Autodesk Fusion 360 part; units mm, degrees
sketch "Sketch1" plane through (0, 0, 0) normal (0, 0, 1) x (1, 0, 0)
  line L0 (0, 0) -> (7, 0)
  line L1 (7, 0) -> (7, 7)
  line L2 (7, 7) -> (0, 7)
  line L3 (0, 7) -> (0, 0)
  line L4 (7, 0) -> (29.8, 0)
  line L5 (29.8, 0) -> (29.8, 7)
  line L6 (29.8, 7) -> (7, 7)
  line L7 (7, 7) -> (7, 0)
  line L8 (29.8, 0) -> (36.8, 0)
  line L9 (36.8, 0) -> (36.8, 7)
  line L10 (36.8, 7) -> (29.8, 7)
  line L11 (29.8, 7) -> (29.8, 0)
  line L12 (0, 7) -> (7, 0)
  line L13 (0, 0) -> (7, 7)
  line L14 (29.8, 7) -> (36.8, 0)
  line L15 (29.8, 0) -> (36.8, 7)
  circle A0 centre (3.5, 3.5) radius 2.3
  circle A1 centre (33.3, 3.5) radius 2.3
  circle A2 centre (3.5, 3.5) radius 3.5
  circle A3 centre (33.3, 3.5) radius 3.5128
  circle A4 centre (33.3, 3.5) radius 3
  circle A5 centre (3.5, 3.5) radius 3
  line L16 (29.8, 7) -> (7, 0)
  line L17 (29.8, 0) -> (7, 7)
  line L18 (7.9, 1) -> (28.9, 1)
  line L19 (28.9, 1) -> (28.9, 6)
  line L20 (28.9, 6) -> (7.9, 6)
  line L21 (7.9, 6) -> (7.9, 1)
  line L22 (7.9, 1) -> (28.9, 6) construction
  line L23 (28.9, 1) -> (7.9, 6) construction
  point P0 (18.4, 3.5)
  dimension "d1" = 7
  dimension "d2" = 7
  dimension "d3" = 22.8
  dimension "d4" = 7
  dimension "d5" = 4.6
  dimension "d6" = 4.6
  dimension "d9" = 6
  dimension "d10" = 6
  dimension "d13" = 21
  dimension "d14" = 5
extrude "Extrude1" add sketch "Sketch1" along normal blind 5 contours L0 L12 A2 | L12 L13 A2 A5 | L12 L13 A2 A5 | L1 L7 L12 A2 | L4 L16 L17 L18 | L1 L7 L16 L17 L18 L20 L21 | L12 L13 A2 A5 | L12 L13 A2 A5 | L12 L13 A0 A5 | L12 L13 A0 A5 | L1 L7 L13 A2 | L5 L11 A3 L16 L17 L18 L19 L20 | L8 L15 A3 | L5 L11 L15 A3 | L16 L17 L18 L20 L21 | L16 L17 L18 | L12 L13 A0 A5 | L2 L13 A2 | L12 L13 A0 A5 | L6 L16 L17 L20 | L5 L11 L14 L15 A3 A4 | L8 L14 L15 A3 A4 | L16 L17 L18 L19 L20 | L16 L17 L20 | L5 L11 L14 A3 | L10 L14 A3 | L14 L15 A1 A4 | L14 L15 A1 A4 | L10 L14 L15 A3 A4 | L9 L14 L15 A3 A4 | L14 L15 A1 A4 | L14 L15 A1 A4
extrude "Extrude2" cut sketch "Sketch1" along normal blind 3.5 contours L12 L13 A0 A5 | L12 L13 A0 A5 | L12 L13 A0 A5 | L12 L13 A0 A5 | L14 L15 A1 A4 | L14 L15 A1 A4 | L14 L15 A1 A4 | L14 L15 A1 A4
extrude "Extrude3" add sketch "Sketch1" along normal blind 8 contours L16 L17 L18 L20 L21 | L16 L17 L18 | L16 L17 L18 L19 L20 | L16 L17 L20
fillet "Fillet1" radius 1.5 1 edges at (7.9, 6, 6.5)
fillet "Fillet2" radius 1.5 1 edges at (7.9, 1, 6.5)
fillet "Fillet3" radius 1.5 1 edges at (28.9, 6, 6.5)
fillet "Fillet4" radius 1.5 1 edges at (28.9, 1, 6.5)
Source: CAD feature listing. Evaluate the final solid. Frame: model axes, mm. A direction names the side the tool comes from. Give positions to 0.01 mm unless a question says otherwise; leave off trailing zeros. Loops run counter-clockwise (first coordinate to the right, second up) from the corner with the lowest first, then second, coordinate; pieces in that order, holes last. Notation, with made-up numbers: (48.25, 32) -> (78.25, 32) arc R27 cw to (78.25, 52) -> close; hole circle Ø1 at (-8, -20.5). An arc over 180 degrees is marked (long way). Use a Markdown table: item, result. Add a question column.
1) Section query B-B, the plane z = 0.75. Return the cut outline in (x, y).
2) Pull-direction query (Y, two-part tool) for faces 1 (the face through (28.45, 1.43, 6.52)), 2 (the face through (35.76, 6.01, 2.46)), 3 (the face through (35.425, 4.381, 4.24)), 4 (the face through (7.9, 4, 6)); classes: +Y half, -Y half, draft (parallel to the pull), parting line (faces both ways), or undercut.
3) Section query D-D, the plane x = 18.5. Return the cut outline in (y, z).
4) Section query C-C, the plane y = 5.25. Return the cut outline in (x, z), then the cut area to 3 significant figures.
5) First-contact query: pin 1 (3.5 mm diameter, centred on x = 3.5, y = 3.5, fed in from -Z); pin 2 (2.5 mm diameter, centred on x = 20, z = 7, fed in from +Y); pin 3 (0.9 mm diameter, centred on x = 21, z = 7, fed in from -Y); pin 4 (1.6 mm diameter, centred on y = 3.5, z = 6, fed in from +X). Flat tips, straight axial feed; report the tip coordinate or a pass-through.
6) Reachability of faces 5 (the face through (0.5, 3.4, 1.7)), 6 (the face through (28.47, 5.55, 6.52)), 7 (the face through (8.33, 1.45, 6.52)), 8 (the face through (8.35, 5.57, 6.52)) from +Z, -Z, +X, -X, +Y, -Y: full face, straight path, thin tool, end or side. Return the list, or none.
7) Section query A-A, the plane x = 5. Return the cut outline in (y, z).
8) Line query: line 1 along Y through (x, z) = (3.5, 1.4); line 2 along X through (y, z) = (1.25, 3); line 3 along X through (y, z) = (1, 1). Output: solid intervals per line, ascending. Write a range as [from, to].
Numbers:
| question | item | result |
|---|---|---|
| 1 | outline | (3.5, 0) -> (33.6, 0) arc R3.51 ccw to (36.8, 3.2) -> (36.8, 3.8) arc R3.51 ccw to (33.6, 7) -> (3.5, 7) arc R3.5 ccw to start; hole circle Ø6 at (3.5, 3.5); hole (29.8, 3.2) -> (29.8, 3.8) arc R3.51 ccw to start; hole circle Ø6 at (33.3, 3.5) |
| 2 | face 1 | -Y half |
| 2 | face 2 | +Y half |
| 2 | face 3 | undercut |
| 2 | face 4 | draft |
| 3 | outline | (0, 0) -> (7, 0) -> (7, 5) -> (6, 5) -> (6, 8) -> (1, 8) -> (1, 5) -> (0, 5) -> close |
| 4 | outline | (0.47, 0) -> (1.06, 0) -> (1.06, 3.5) -> (2.01, 3.5) -> (2.01, 5) -> (0.47, 5) -> close; (4.99, 3.5) -> (5.94, 3.5) -> (5.94, 0) -> (30.86, 0) -> (30.86, 3.5) -> (31.81, 3.5) -> (31.81, 5) -> (28.7, 5) -> (28.7, 8) -> (8.1, 8) -> (8.1, 5) -> (4.99, 5) -> close; (34.79, 3.5) -> (35.74, 3.5) -> (35.74, 0) -> (36.35, 0) -> (36.35, 5) -> (34.79, 5) -> close |
| 4 | area | 198 mm2 |
| 5 | pin 1 | passes through |
| 5 | pin 2 | stops at y = 6 |
| 5 | pin 3 | stops at y = 1 |
| 5 | pin 4 | stops at x = 28.9 |
| 6 | face 5 | -Z |
| 6 | face 6 | +Z, +X, +Y |
| 6 | face 7 | +Z, -X, -Y |
| 6 | face 8 | +Z, -X, +Y |
| 7 | outline | (0, 0) -> (0.9, 0) -> (0.9, 3.5) -> (1.76, 3.5) -> (1.76, 5) -> (0, 5) -> close; (5.24, 3.5) -> (6.1, 3.5) -> (6.1, 0) -> (7, 0) -> (7, 5) -> (5.24, 5) -> close |
| 8 | line 1 | y = [0, 0.5], [6.5, 7] |
| 8 | line 2 | x = [0.82, 1.52], [5.48, 31.32], [35.28, 36] |
| 8 | line 3 | x = [1.05, 1.84], [5.16, 31.64], [34.96, 35.77] |
